```python
from build123d import *

# Parameters (mm, degrees)
SKETCH_1_W                       = 4
SKETCH_1_H                       = 4
EXTRUDE_1_DEPTH                  = 98.5
FILLET_1_R                       = 1
FILLET_2_R                       = 2
FILLET_3_R                       = 0.5
PATTERN_CIRCULAR_1_COUNT         = 4
FILLET_1_OF_PATTERN_CIRCULAR_1_R = 1
FILLET_2_OF_PATTERN_CIRCULAR_1_R = 2
FILLET_3_OF_PATTERN_CIRCULAR_1_R = 0.5
SKETCH_2_R                       = 3.4
CUT_EXTRUDE_1_DEPTH              = 99.5


with BuildPart() as part:
    # 草图1 → 凸台-拉伸1 (new body)
    with BuildSketch(Plane.XY):
        Polygon((5.7, 0), (5.7, 4.427207794), (9.672792206, 8.4), (13.2, 8.4), (13.2, 4.1), (14.1, 4.1), (14.1, 5.1), (15, 5.1), (15, 15), (5.1, 15), (5.1, 14.1), (4.1, 14.1), (4.1, 13.2), (8.4, 13.2), (8.4, 9.672792206), (4.427207794, 5.7), (0, 5.7), (0, 0), align=None)
        with Locations((11.7, 11.7)):
            Rectangle(SKETCH_1_W, SKETCH_1_H, mode=Mode.SUBTRACT)
    extrude_1 = extrude(amount=EXTRUDE_1_DEPTH)

    # 圆角1
    fillet_1_edges = [part.edges().sort_by_distance(p)[0] for p in [
        (13.7, 9.7, 49.25),
        (13.7, 13.7, 49.25),
        (9.7, 13.7, 49.25),
        (9.7, 9.7, 49.25),
    ]]
    fillet(fillet_1_edges, radius=FILLET_1_R)

    # 圆角2
    fillet_2_edges = [part.edges().sort_by_distance(p)[0] for p in [
        (15, 15, 49.25),
    ]]
    fillet(fillet_2_edges, radius=FILLET_2_R)

    # 圆角3
    fillet_3_edges = [part.edges().sort_by_distance(p)[0] for p in [
        (4.427207794, 5.7, 49.25),
        (8.4, 9.672792206, 49.25),
        (8.4, 13.2, 49.25),
        (13.2, 8.4, 49.25),
        (9.672792206, 8.4, 49.25),
        (5.7, 4.427207794, 49.25),
    ]]
    fillet(fillet_3_edges, radius=FILLET_3_R)

    # 阵列(圆周)1: 凸台-拉伸1 ×4 about axis
    pattern_circular_1_axis = Axis((0, 0, 0), (0, 0, 1))
    for i in range(1, PATTERN_CIRCULAR_1_COUNT):
        add(extrude_1.rotate(pattern_circular_1_axis, i * 360 / PATTERN_CIRCULAR_1_COUNT))

    # 圆角1 of 阵列(圆周)1
    fillet_1_of_pattern_circular_1_edges = [part.edges().sort_by_distance(p)[0] for p in [
        (-9.7, 13.7, 49.25),
        (-13.7, 13.7, 49.25),
        (-13.7, 9.7, 49.25),
        (-9.7, 9.7, 49.25),
        (-13.7, -9.7, 49.25),
        (-13.7, -13.7, 49.25),
        (-9.7, -13.7, 49.25),
        (-9.7, -9.7, 49.25),
        (9.7, -13.7, 49.25),
        (13.7, -13.7, 49.25),
        (13.7, -9.7, 49.25),
        (9.7, -9.7, 49.25),
    ]]
    fillet(fillet_1_of_pattern_circular_1_edges, radius=FILLET_1_OF_PATTERN_CIRCULAR_1_R)

    # 圆角2 of 阵列(圆周)1
    fillet_2_of_pattern_circular_1_edges = [part.edges().sort_by_distance(p)[0] for p in [
        (-15, 15, 49.25),
        (-15, -15, 49.25),
        (15, -15, 49.25),
    ]]
    fillet(fillet_2_of_pattern_circular_1_edges, radius=FILLET_2_OF_PATTERN_CIRCULAR_1_R)

    # 圆角3 of 阵列(圆周)1
    fillet_3_of_pattern_circular_1_edges = [part.edges().sort_by_distance(p)[0] for p in [
        (-5.7, 4.427207794, 49.25),
        (-9.672792206, 8.4, 49.25),
        (-13.2, 8.4, 49.25),
        (-8.4, 13.2, 49.25),
        (-8.4, 9.672792206, 49.25),
        (-4.427207794, 5.7, 49.25),
        (-4.427207794, -5.7, 49.25),
        (-8.4, -9.672792206, 49.25),
        (-8.4, -13.2, 49.25),
        (-13.2, -8.4, 49.25),
        (-9.672792206, -8.4, 49.25),
        (-5.7, -4.427207794, 49.25),
        (5.7, -4.427207794, 49.25),
        (9.672792206, -8.4, 49.25),
        (13.2, -8.4, 49.25),
        (8.4, -13.2, 49.25),
        (8.4, -9.672792206, 49.25),
        (4.427207794, -5.7, 49.25),
    ]]
    fillet(fillet_3_of_pattern_circular_1_edges, radius=FILLET_3_OF_PATTERN_CIRCULAR_1_R)

    # 草图2 → 切除-拉伸1 (cut, through all)
    with BuildSketch(Plane.XY.offset(98.5)):
        Circle(SKETCH_2_R)
    extrude(amount=-CUT_EXTRUDE_1_DEPTH, mode=Mode.SUBTRACT)


solid = part.part
```
Could you check a few things on this model? Use its own coordinates, in mm. A direction names the side the tool comes from. Round coordinates to 2 decimals unless told otherwise and drop trailing zeros. Loops run counter-clockwise (first coordinate to the right, second up) from the corner with the lowest first, then second, coordinate; pieces in that order, holes last. Notation, with made-up numbers: M 24.25,77.25 L 74.25,77.25 A15 ccw 74.25,101.25 Z; hole C 3,43.5 d8. An arc over 180 degrees is marked long. Put each result on its own line as item: value.
Q1. On a 3-axis mill with a long thin cutter (end or side, diameter ignored), from which of +Z, -Z, +X, -X, +Y, -Y can I reach the whole of each face in a straight line? I mean faces 1 (the face through (-12, -9.7, 49)), 2 (the face through (1.2, 3.4, 98.5)). Say none if no direction works.
Check result:
face 1: +Z, -Z
face 2: +Z, +X, -X, +Y, -Y
Q2. Imagine slicing it at A-A (x = 0). Write out the boundary of the cut face in (y, z).
Check result:
outline: M -5.7,0 L -3.4,0 L -3.4,98.5 L -5.7,98.5 Z; M 3.4,0 L 5.7,0 L 5.7,98.5 L 3.4,98.5 Z
Q3. Thinking about a two-plate mould opening in Y: for faces 3 (the face through (9, -15, 49)), 4 (the face through (-11, 8.4, 49)), 5 (the face through (15, -9, 49)), which applies, released by +Y, released by -Y, zero draft, split by the parting line, or undercut?
Check result:
face 3: released by -Y
face 4: undercut
face 5: zero draft
Q4. For pin 1 (3 mm diameter, centred on x = 2, z = 69, fed in from +Y); pin 2 (0.8 mm diameter, centred on x = 4.5, z = 26, fed in from +Y); pin 3 (4 mm diameter, centred on y = -2.5, z = 65.5, fed in from +X), each with a flat end and sliding along its axis, tell me the tip position at first contact or that it passes through.
Check result:
pin 1: y = 5.7
pin 2: y = 14.1
pin 3: x = 14.1
Q5. I need wall thicknesses on probe 1 along Y at (x, z) = (12.25, 54); probe 2 along Y at (x, z) = (0, 32.5). Which ranges of each line are inside material? Lowest first, please.
Check result:
probe 1: -15 to -13.7, -9.7 to -8.4, 8.4 to 9.7, 13.7 to 15
probe 2: -5.7 to -3.4, 3.4 to 5.7
Q6. Imagine slicing it at B-B (y = 2). Write out the boundary of the cut face in (x, z).
Check result:
outline: M -5.7,0 L -2.75,0 L -2.75,98.5 L -5.7,98.5 Z; M 2.75,0 L 5.7,0 L 5.7,98.5 L 2.75,98.5 Z
Q7. Imagine slicing it at C-C (z = 89). State how many separate pieces and enclosed holes the cut face has, then the cut area to 3 significant figures.
Check result:
separate pieces: 1
enclosed holes: 5
area: 293 mm2
